from build123d import *

# Parameters (mm, degrees)
SKETCH001_R  = 18
POCKET_DEPTH = 14.9


with BuildPart() as part:
    # Sketch → Revolution (revolve)
    with BuildSketch(Plane.XZ):
        Polygon((10, 0), (8.75, 0.721688), (8.75, 14.178312), (10, 14.9), (14.9, 14.9), (18, 13.110214), (18, 1.789786), (14.9, 0), align=None)
    revolve(axis=Axis((0, 0, 0), (0, 0, 1)))

    # Sketch001 → Pocket (cut)
    with BuildSketch(Plane(origin=(0, 0, 14.9), x_dir=(-1, 0, 0), z_dir=(0, 0, 1))):
        Circle(SKETCH001_R)
        Polygon((-15, 8.660254), (-15, -8.660254), (0, -17.320508), (15, -8.660254), (15, 8.660254), (0, 17.320508), align=None, mode=Mode.SUBTRACT)
    extrude(amount=-POCKET_DEPTH, mode=Mode.SUBTRACT)


solid = part.part
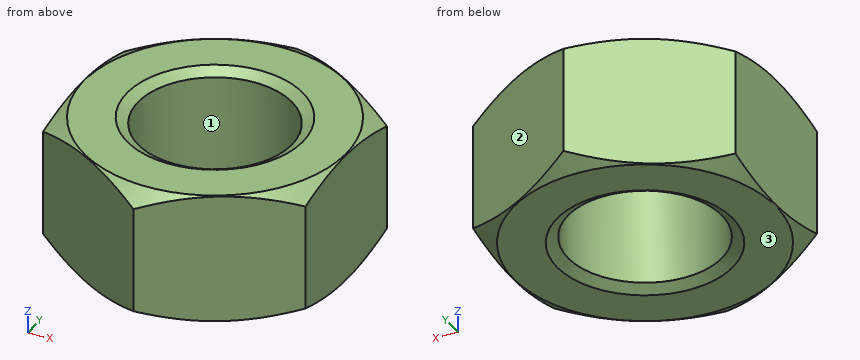
Check sheet for the modelled part. Datum: model origin and axes. Units: mm. Face numbers are marked on the shaded views. Give positions to 0.01 mm unless a question says otherwise; leave off trailing zeros. Write each loop counter-clockwise with the first axis right and the second up, starting at its lowest first coordinate (ties: lowest second). Pieces come first, ordered by that corner, then holes. Notation, with made-up numbers: (34, 48) -> (38, 48) arc R29 cw to (38, 72) -> close; hole circle Ø8 at (67.25, -22). An arc over 180 degrees is marked (long way). Use one line per item in the form item = value. Start each with the question number.
1. Go/stop test with flat-tipped pins: P1, Ø12, axis at x = 4, y = 6.5, coming from the +Z side; P2, Ø3, axis at y = -13, z = 11.5, coming from the -X side; P3, Ø2, axis at x = 10.5, z = 3, coming from the -Y side; P4, Ø1.5, axis at y = -12.5, z = 5, coming from the -X side. Record where each tip stops, or that it passes through.
2. Mould release check, pull along X, two halves, no side actions. Record for the marked faces 1, 2 and 3: pulls with the +X half, pulls with the -X half, needs draft (parallel to the pull), parting line crosses it, or undercut.
3. Section check A-A (z = 8). Record the cut outline in (x, y), and give its area (3 significant figures).
4. Thickness scan on line 1 along Y through (x, z) = (0, 9.25); line 2 along X through (y, z) = (4.5, 5.5); line 3 along X through (y, z) = (1, 5). Record the ranges inside material, lowest first. Write a range as from..to.
5. Section check B-B (y = 0). Record the cut outline in (x, z).
Conclusion:
q1.P1 = 14.9
q1.P2 = -10.08
q1.P3 = -11.84
q1.P4 = -9.65
q2.face_1 = undercut
q2.face_2 = pulls with the +X half
q2.face_3 = needs draft
q3.outline = (-15, -8.66) -> (0, -17.32) -> (15, -8.66) -> (15, 8.66) -> (0, 17.32) -> (-15, 8.66) -> close; hole circle Ø17.5 at (0, 0)
q3.area = 539 mm²
q4.line_1 = -17.32..-8.75, 8.75..17.32
q4.line_2 = -15..-7.5, 7.5..15
q4.line_3 = -15..-8.69, 8.69..15
q5.outline = (-15, 0.06) -> (-14.9, 0) -> (-10, 0) -> (-8.75, 0.72) -> (-8.75, 14.18) -> (-10, 14.9) -> (-14.9, 14.9) -> (-15, 14.84) -> close; (8.75, 0.72) -> (10, 0) -> (14.9, 0) -> (15, 0.06) -> (15, 14.84) -> (14.9, 14.9) -> (10, 14.9) -> (8.75, 14.18) -> close
